For this review, take the finished solid that the model builds, in its own axes (mm). Coordinates: 2 decimals unless noted, no trailing zeros. Loops run counter-clockwise (first coordinate to the right, second up) from the corner with the lowest first, then second, coordinate; pieces in that order, holes last. Notation, with made-up numbers: (19.25, 3.5) -> (71.25, 3.5) arc R24 cw to (71.25, 30.5) -> close; hole circle Ø11 at (-5.75, -24). An arc over 180 degrees is marked (long way). Answer in a Markdown table with one row per item.
from build123d import *

# Parameters (mm, degrees)
SKETCH_2_W               = 20
SKETCH_2_H               = 30
EXTRUDE_3_DEPTH          = 30
SKETCH_4_W               = 8
SKETCH_4_H               = 2
CUT_EXTRUDE_1_DEPTH      = 20
CUT_EXTRUDE_6_DEPTH      = 67.759624542
CUT_EXTRUDE_6_DEPTH_BACK = 5
CUT_EXTRUDE_7_DEPTH      = 5


with BuildPart() as part:
    # 草图2 → 凸台-拉伸3 (new body)
    with BuildSketch(Plane.XY):
        with Locations((-41.544616295, 10.663270327)):
            Rectangle(SKETCH_2_W, SKETCH_2_H)
    extrude(amount=EXTRUDE_3_DEPTH)

    # 草图4 → 切除-拉伸1 (cut)
    with BuildSketch(Plane(origin=(0, 0.663270327, 0), x_dir=(-1, 0, 0), z_dir=(0, -1, 0))):
        with Locations((31.544616295, -15)):
            Rectangle(SKETCH_4_W, SKETCH_4_H)
    extrude(amount=-CUT_EXTRUDE_1_DEPTH, mode=Mode.SUBTRACT)

    # 草图5 → 切除-拉伸6 (cut, two sides: drawn at the far end of the back side and taken through both)
    with BuildSketch(Plane.XZ.offset(4.336729673).offset(-CUT_EXTRUDE_6_DEPTH_BACK)):
        with BuildLine():
            Line((-34.594616295, 15), (-32.494616295, 15))
            ThreePointArc((-32.494616295, 15), (-33.544616295, 16.05), (-34.594616295, 15))
        make_face()
        with BuildLine():
            Line((-33.864772507, 14), (-33.224460083, 14))
            ThreePointArc((-33.224460083, 14), (-32.696481865, 14.380994355), (-32.494616295, 15))
            Line((-32.494616295, 15), (-34.594616295, 15))
            ThreePointArc((-34.594616295, 15), (-34.392750725, 14.380994355), (-33.864772507, 14))
        make_face()
        with BuildLine():
            ThreePointArc((-33.864772507, 14), (-33.544616295, 13.95), (-33.224460083, 14))
            Line((-33.224460083, 14), (-33.864772507, 14))
        make_face()
    extrude(amount=CUT_EXTRUDE_6_DEPTH + CUT_EXTRUDE_6_DEPTH_BACK, mode=Mode.SUBTRACT)

    # 草图7 → 切除-拉伸7 (cut)
    with BuildSketch(Plane(origin=(0, 25.663270327, 0), x_dir=(1, 0, 0), z_dir=(0, 1, 0))):
        with BuildLine():
            ThreePointArc((-32.494616295, -15), (-33.544616295, -13.95), (-34.594616295, -15))
            Line((-34.594616295, -15), (-32.494616295, -15))
        make_face()
        with BuildLine():
            Line((-32.494616295, -15), (-34.594616295, -15))
            ThreePointArc((-34.594616295, -15), (-33.544616295, -16.05), (-32.494616295, -15))
        make_face()
    extrude(amount=-CUT_EXTRUDE_7_DEPTH, mode=Mode.SUBTRACT)


solid = part.part
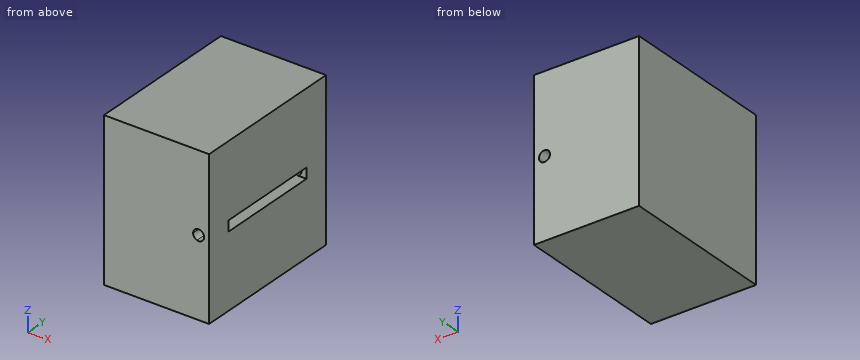
Item 1: Take a section at A-A, the plane z = 14.5. State the section outline as (x, y) points.
Worked answers:
| item | result |
|---|---|
| outline | (-51.54, -4.34) -> (-34.47, -4.34) -> (-34.47, 0.66) -> (-35.54, 0.66) -> (-35.54, 20.66) -> (-34.47, 20.66) -> (-34.47, 25.66) -> (-51.54, 25.66) -> close; (-32.62, -4.34) -> (-31.54, -4.34) -> (-31.54, 0.66) -> (-32.62, 0.66) -> close; (-32.62, 20.66) -> (-31.54, 20.66) -> (-31.54, 25.66) -> (-32.62, 25.66) -> close |
Item 2: Insertion check: pin 1 (1.7 mm diameter, centred on x = -33.54, z = 15, fed in from +Y); pin 2 (0.5 mm diameter, centred on x = -34.5, z = 15, fed in from +Y). Each pin has a flat end and moves straight along its axis. Give the tip position at first contact, or say it passes through.
Worked answers:
| item | result |
|---|---|
| pin 1 | through |
| pin 2 | y = 25.66 |
Item 3: For L1, parallel to Z at x = -34, y = 19.5; L2, parallel to X at y = 24.6, z = 15, list the stretches that pass through material, from the lowest coordinate up.
Worked answers:
| item | result |
|---|---|
| L1 | 0 to 14, 16 to 30 |
| L2 | -51.54 to -34.59, -32.49 to -31.54 |
